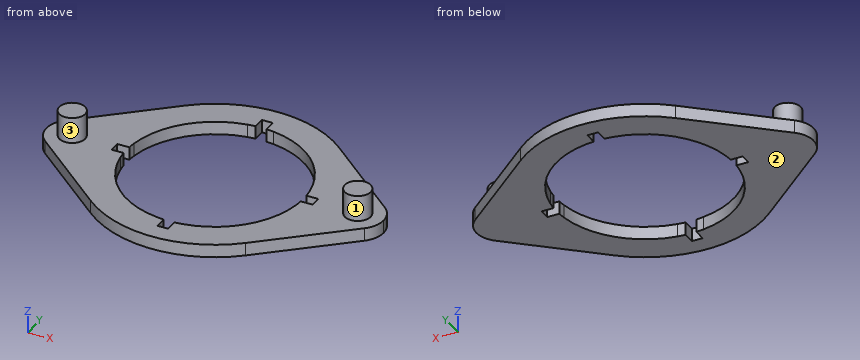
```python
from build123d import *

# Parameters (mm, degrees)
F0_R     = 3
F1_DEPTH = 3
F2_DEPTH = 9


with BuildPart() as f1:
    # F0 (on Top) → F1 (new body)
    with BuildSketch(Plane.XY):
        with BuildLine():
            ThreePointArc((27.4128787879, -2.1872532), (27, 0), (27.4128787879, 2.1872532))
            ThreePointArc((27.4128787879, 2.1872532), (24.5129138593, 12.4646321295), (17.916666852, 20.8624794527))
            ThreePointArc((17.916666852, 20.8624794527), (2.047e-07, 27.5), (-17.9166665414, 20.8624797195))
            ThreePointArc((-17.9166665414, 20.8624797195), (-24.5129137666, 12.464632312), (-27.4128787879, 2.1872532))
            ThreePointArc((-27.4128787879, 2.1872532), (-27.1041231665, 1.1129404133), (-27, 0))
            ThreePointArc((-27, 0), (-27.1041231665, -1.1129404133), (-27.4128787879, -2.1872532))
            ThreePointArc((-27.4128787879, -2.1872532), (-24.5129136468, -12.4646325475), (-17.9166661404, -20.8624800638))
            ThreePointArc((-17.9166661404, -20.8624800638), (2.794e-07, -27.5), (17.9166665643, -20.8624796998))
            ThreePointArc((17.9166665643, -20.8624796998), (24.5129137734, -12.4646322985), (27.4128787879, -2.1872532))
        make_face()
        with BuildLine():
            ThreePointArc((3, 20.2792997907), (14.4956890143, 14.4956890143), (20.2792997907, 3))
            Line((20.2792997907, 3), (25, 3))
            Line((25, 3), (25, -3))
            Line((25, -3), (20.2792997907, -3))
            ThreePointArc((20.2792997907, -3), (14.4956890143, -14.4956890143), (3, -20.2792997907))
            Line((3, -20.2792997907), (3, -25))
            Line((3, -25), (-3, -25))
            Line((-3, -25), (-3, -20.2792997907))
            ThreePointArc((-3, -20.2792997907), (-14.4956890143, -14.4956890143), (-20.2792997907, -3))
            Line((-20.2792997907, -3), (-25, -3))
            Line((-25, -3), (-25, 3))
            Line((-25, 3), (-20.2792997907, 3))
            ThreePointArc((-20.2792997907, 3), (-14.4956890143, 14.4956890143), (-3, 20.2792997907))
            Line((-3, 20.2792997907), (-3, 25))
            Line((-3, 25), (3, 25))
            Line((3, 25), (3, 20.2792997907))
        make_face(mode=Mode.SUBTRACT)
        with BuildLine():
            ThreePointArc((-27.4128787879, 2.1872532), (-24.5129137666, 12.464632312), (-17.9166665414, 20.8624797195))
            Line((-17.9166665414, 20.8624797195), (-36.9090909114, 4.5518137315))
            ThreePointArc((-36.9090909114, 4.5518137315), (-31.5502644899, 5.8222218225), (-27.4128787879, 2.1872532))
        make_face()
        with BuildLine():
            ThreePointArc((-27.4128787879, -2.1872532), (-27.5, 0), (-27.4128787879, 2.1872532))
            ThreePointArc((-27.4128787879, 2.1872532), (-31.5502644899, 5.8222218225), (-36.9090909114, 4.5518137315))
            ThreePointArc((-36.9090909114, 4.5518137315), (-39, 5.6e-09), (-36.9090909199, -4.5518137242))
            ThreePointArc((-36.9090909199, -4.5518137242), (-31.5502644953, -5.8222218239), (-27.4128787879, -2.1872532))
        make_face()
        with Locations((-33, 0)):
            Circle(F0_R, mode=Mode.SUBTRACT)
        with Locations((-33, 0)):
            Circle(F0_R)
        with BuildLine():
            Line((-36.9090909199, -4.5518137242), (-17.9166661404, -20.8624800638))
            ThreePointArc((-17.9166661404, -20.8624800638), (-24.5129136468, -12.4646325475), (-27.4128787879, -2.1872532))
            ThreePointArc((-27.4128787879, -2.1872532), (-31.5502644953, -5.8222218239), (-36.9090909199, -4.5518137242))
        make_face()
        with BuildLine():
            ThreePointArc((27.4128787879, 2.1872532), (27.478211065, 1.0944937947), (27.5, 0))
            ThreePointArc((27.5, 0), (27.478211065, -1.0944937947), (27.4128787879, -2.1872532))
            ThreePointArc((27.4128787879, -2.1872532), (31.5502644944, -5.8222218236), (36.9090909184, -4.5518137255))
            ThreePointArc((36.9090909184, -4.5518137255), (38.4522722562, -2.5045413242), (39, 0))
            ThreePointArc((39, 0), (38.4522722545, 2.5045413278), (36.9090909125, 4.5518137306))
            ThreePointArc((36.9090909125, 4.5518137306), (31.5502644906, 5.8222218227), (27.4128787879, 2.1872532))
        make_face()
        with Locations((33, 0)):
            Circle(F0_R, mode=Mode.SUBTRACT)
        with Locations((33, 0)):
            Circle(F0_R)
        with BuildLine():
            ThreePointArc((36.9090909184, -4.5518137255), (31.5502644944, -5.8222218236), (27.4128787879, -2.1872532))
            ThreePointArc((27.4128787879, -2.1872532), (24.5129137734, -12.4646322985), (17.9166665643, -20.8624796998))
            Line((17.9166665643, -20.8624796998), (36.9090909184, -4.5518137255))
        make_face()
        with BuildLine():
            ThreePointArc((17.916666852, 20.8624794527), (24.5129138593, 12.4646321295), (27.4128787879, 2.1872532))
            ThreePointArc((27.4128787879, 2.1872532), (31.5502644906, 5.8222218227), (36.9090909125, 4.5518137306))
            Line((36.9090909125, 4.5518137306), (17.916666852, 20.8624794527))
        make_face()
        with BuildLine():
            ThreePointArc((27.4128787879, -2.1872532), (27.478211065, -1.0944937947), (27.5, 0))
            ThreePointArc((27.5, 0), (27.478211065, 1.0944937947), (27.4128787879, 2.1872532))
            ThreePointArc((27.4128787879, 2.1872532), (27, 0), (27.4128787879, -2.1872532))
        make_face()
        with BuildLine():
            ThreePointArc((-27, 0), (-27.1041231665, 1.1129404133), (-27.4128787879, 2.1872532))
            ThreePointArc((-27.4128787879, 2.1872532), (-27.5, 0), (-27.4128787879, -2.1872532))
            ThreePointArc((-27.4128787879, -2.1872532), (-27.1041231665, -1.1129404133), (-27, 0))
        make_face()
        with BuildLine():
            ThreePointArc((1.25, 20.4618547546), (2.126959468, 20.3893610351), (3, 20.2792997907))
            Line((3, 20.2792997907), (3, 25))
            Line((3, 25), (-3, 25))
            Line((-3, 25), (-3, 20.2792997907))
            ThreePointArc((-3, 20.2792997907), (-2.126959468, 20.3893610351), (-1.25, 20.4618547546))
            Line((-1.25, 20.4618547546), (-1.25, 23.25))
            Line((-1.25, 23.25), (1.25, 23.25))
            Line((1.25, 23.25), (1.25, 20.4618547546))
        make_face()
        with BuildLine():
            Line((-23.25, 1.25), (-20.4618547546, 1.25))
            ThreePointArc((-20.4618547546, 1.25), (-20.3893610351, 2.126959468), (-20.2792997907, 3))
            Line((-20.2792997907, 3), (-25, 3))
            Line((-25, 3), (-25, -3))
            Line((-25, -3), (-20.2792997907, -3))
            ThreePointArc((-20.2792997907, -3), (-20.3893610351, -2.126959468), (-20.4618547546, -1.25))
            Line((-20.4618547546, -1.25), (-23.25, -1.25))
            Line((-23.25, -1.25), (-23.25, 1.25))
        make_face()
        with BuildLine():
            Line((3, -25), (3, -20.2792997907))
            ThreePointArc((3, -20.2792997907), (2.126959468, -20.3893610351), (1.25, -20.4618547546))
            Line((1.25, -20.4618547546), (1.25, -23.25))
            Line((1.25, -23.25), (-1.25, -23.25))
            Line((-1.25, -23.25), (-1.25, -20.4618547546))
            ThreePointArc((-1.25, -20.4618547546), (-2.126959468, -20.3893610351), (-3, -20.2792997907))
            Line((-3, -20.2792997907), (-3, -25))
            Line((-3, -25), (3, -25))
        make_face()
        with BuildLine():
            ThreePointArc((20.2792997907, 3), (20.3893610351, 2.126959468), (20.4618547546, 1.25))
            Line((20.4618547546, 1.25), (23.25, 1.25))
            Line((23.25, 1.25), (23.25, -1.25))
            Line((23.25, -1.25), (20.4618547546, -1.25))
            ThreePointArc((20.4618547546, -1.25), (20.3893610351, -2.126959468), (20.2792997907, -3))
            Line((20.2792997907, -3), (25, -3))
            Line((25, -3), (25, 3))
            Line((25, 3), (20.2792997907, 3))
        make_face()
    extrude(amount=F1_DEPTH)

    # F0 (on Top) → F2 (join)
    with BuildSketch(Plane.XY):
        with Locations((-33, 0)):
            Circle(F0_R)
        with Locations((33, 0)):
            Circle(F0_R)
    extrude(amount=F2_DEPTH)


solid = f1.part
```
Source: CAD feature listing. Evaluate the final solid. Frame: model axes, mm. Face numbers are marked on the shaded views. Round coordinates to 2 decimals unless told otherwise and drop trailing zeros. Loops run counter-clockwise (first coordinate to the right, second up) from the corner with the lowest first, then second, coordinate; pieces in that order, holes last.
1. Ray query, L1, parallel to X at y = 1.5, z = 3.25; L2, parallel to Z at x = -5.5, y = -22.5; L3, parallel to Y at x = 7, z = 1. Return the intervals inside material, ascending.
2. Section query A-A on x = 17. Output: boundary loops of the cut face in (y, z), and give its area (3 significant figures).
3. Section query B-B on y = -12. Output: boundary loops of the cut face in (x, z).
4. Section query D-D on x = 33. Output: boundary loops of the cut face in (y, z).
5. Contact query for flat-ended pins moving along their axis: pin 1 (2 mm diameter, centred on x = -22.5, z = 1, fed in from +Y); pin 2 (2 mm diameter, centred on y = -22, z = 1.5, fed in from -X); pin 3 (2 mm diameter, centred on y = 21.5, z = 1.5, fed in from +X). Output: stop coordinate, or through.
6. Section query C-C on z = 7. Output: boundary loops of the cut face in (x, y).
7. Mould query, pull axis X, two halves, no side actions, for the marked faces 1, 2 and 3. Classes: released by +X, released by -X, zero draft, split by the parting line, or undercut.
Answers below:
1. L1: x = -35.6 to -30.4, 30.4 to 35.6
1. L2: z = 0 to 3
1. L3: y = -26.59 to -19.27, 19.27 to 26.59
2. outline: (-21.62, 0) - (-11.46, 0) - (-11.46, 3) - (-21.62, 3) - close; (11.46, 0) - (21.62, 0) - (21.62, 3) - (11.46, 3) - close
2. area: 61.0 mm2
3. outline: (-28.24, 0) - (-16.62, 0) - (-16.62, 3) - (-28.24, 3) - close; (16.62, 0) - (28.24, 0) - (28.24, 3) - (16.62, 3) - close
4. outline: (-7.91, 0) - (7.91, 0) - (7.91, 3) - (3, 3) - (3, 9) - (-3, 9) - (-3, 3) - (-7.91, 3) - close
5. pin 1: stops at y = 17.79
5. pin 2: stops at x = -17.76
5. pin 3: stops at x = 18.34
6. outline: circle Ø6 at (-33, 0); circle Ø6 at (33, 0)
7. face 1: undercut
7. face 2: zero draft
7. face 3: undercut
